Can you work these out from the model? Positions are in its coordinate system, mm. Face numbers are marked on the shaded views. A direction names the side the tool comes from. Round coordinates to 2 decimals unless told otherwise and drop trailing zeros. Loops run counter-clockwise (first coordinate to the right, second up) from the corner with the lowest first, then second, coordinate; pieces in that order, holes last.
(1) I want a section at D-D on y = 15. Write out the boundary of the cut face in (x, z), plus the area to 3 significant figures.
(2) Which directions (+Z, -Z, +X, -X, +Y, -Y) give clear straight access to the entire face, cutting with the end or side of a thin tool? Please do the marked faces 4, 5 and 6.
(3) If I drill on line 1 along Z through (x, y) = (14.5, 14.8); line 2 along Z through (x, y) = (9, 11.5); line 3 along X through (y, z) = (15.35, 0), over which ranges is the centre line in solid material (lowest first)?
(4) I want a section at C-C on y = 10.25. Write out the boundary of the cut face in (x, z), plus the area to 3 significant figures.
(5) I want a section at A-A on x = 33.5. Write out the boundary of the cut face in (y, z).
(6) Thinking about a two-plate mould opening in Y: for the marked faces 1, 2 and 3, which applies, released by +Y, released by -Y, zero draft, split by the parting line, or undercut?
(7) Will these pins go through, and if not, where does the flat tip stop? pin 1 Ø1.5 at (y, z) = (20.5, 12.5) entering from -X; pin 2 Ø10 at (y, z) = (7, -0.5) entering from -X; pin 3 Ø3.5 at (y, z) = (16, 0) entering from +X; pin 4 Ø0.6 at (x, z) = (49, -0.5) entering from +Y.
(8) I want a section at B-B on z = -8. Write out the boundary of the cut face in (x, y), plus the area to 3 significant figures.
Autodesk Inventor part; units mm, degrees
ref_plane "YZ Plane" through (0, 0, 0) normal (1, 0, 0) x (0, 1, 0)
ref_plane "XZ Plane" through (0, 0, 0) normal (0, 1, 0) x (-1, 0, 0)
ref_plane "XY Plane" through (0, 0, 0) normal (0, 0, 1) x (1, 0, 0)
sketch "Sketch1" plane through (0, 0, 0) normal (0, 0, 1) x (1, 0, 0)
  line L0 (0, 0) -> (50, 0)
  line L1 (50, 0) -> (50, 8.5)
  arc A0 (50, 8.5) -> (43.9926, 24) centre (27, 8.5) ccw
  line L2 (43.9926, 24) -> (0, 24)
  line L3 (0, 24) -> (0, 0)
  dimension "d3" = 50
  dimension "d4" = 24
  dimension "d5" = 23
  dimension "d6" = 8.5
extrude "Extrusion1" add sketch "Sketch1" along normal mid plane 39
sketch "Sketch2" plane through (0, 0, 0) normal (0, 0, 1) x (1, 0, 0)
  line L0 (0, 0) -> (0, 24)
  line L1 (0, 13.7) -> (38, 13.7)
  arc A0 (38, 5.7) -> (38, 13.7) centre (38, 9.7) ccw
  line L2 (38, 5.7) -> (24, 5.7)
  line L3 (24, 5.7) -> (24, 0)
  line L4 (50, 0) -> (0, 0)
  line L5 (24, 0) -> (0, 0)
  line L6 (0, 0) -> (0, 13.7)
  dimension "d9" = 5.7
  dimension "d10" = 26
  dimension "d11" = 4
  dimension "d12" = 38
extrude "Extrusion2" cut sketch "Sketch2" along normal mid plane 31
sketch "Sketch3" plane through (0, 0, 0) normal (0, 0, 1) x (1, 0, 0)
  line L0 (0, 24) -> (43.9926, 24)
  line L1 (8, 24) -> (8, 18.2)
  line L2 (8, 18.2) -> (22, 18.2)
  line L3 (22, 18.2) -> (22, 0)
  line L4 (50, 0) -> (0, 0)
  line L5 (45, 0) -> (48, 8.5)
  line L6 (48, 8.5) -> (50, 8.5)
  line L7 (50, 8.5) -> (50, 0)
  line L8 (50, 24) -> (50, 8.5)
  line L9 (8, 24) -> (50, 24)
  line L10 (0, 13.7) -> (38, 13.7)
  dimension "d15" = 4.5
  dimension "d16" = 5
  dimension "d17" = 2
  dimension "d19" = 8.5
  dimension "d20" = 42
  dimension "d31" = 28
extrude "Extrusion3" cut sketch "Sketch3" along normal mid plane 13 contours L0 L9 L8 L6 L5 L4 L3 L2 L1
fillet "Fillet1" radius 6.5 2 edges at (8, 21.1, 6.5) (8, 21.1, -6.5)
sketch "Sketch4" plane through (22, 18.2, 6.5) normal (0, 1, 0) x (1, 0, 0)
  arc A0 (-7.5, 13) -> (-7.5, 0) centre (-7.5, 6.5) ccw
  point P0 (-22, 6.5)
hole "Hole1" at (14.5, 18.2, 0) direction (0, -1, 0) diameter 5.2 end through all countersink diameter 9.5 countersink angle 90
chamfer "Chamfer1" distance 4 angle 45 3 edges at (0, 24, 0) (21.9963, 24, -19.5) (21.9963, 24, 19.5)
properties material "Steel, Carbon"
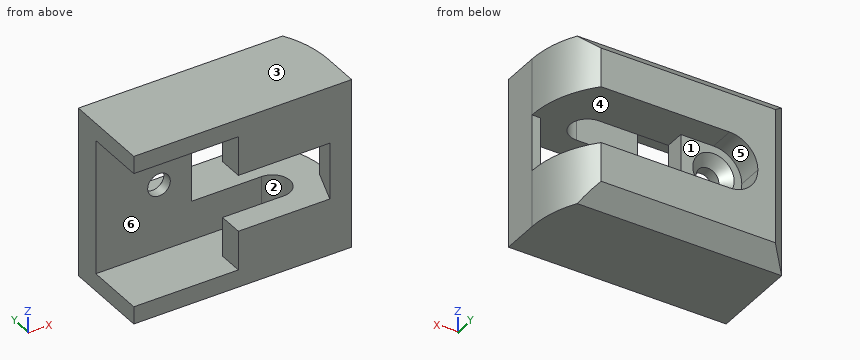
Filled sheet:
1. outline: (0, -19.5) - (49.06, -19.5) - (49.06, -6.5) - (22, -6.5) - (22, 6.5) - (49.06, 6.5) - (49.06, 19.5) - (0, 19.5) - close; hole circle Ø5.2 at (14.5, 0)
1. area: 1,540 mm2
2. face 4: +Y
2. face 5: +X, +Y
2. face 6: -X
3. line 1: z = -19.5 to -2.6, 2.6 to 19.5
3. line 2: z = -19.5 to -15.5, 15.5 to 19.5
3. line 3: x = 0 to 11.9, 17.1 to 22
4. outline: (0, -19.5) - (49.93, -19.5) - (49.93, -6.5) - (41.96, -6.5) - (41.96, -15.5) - (0, -15.5) - close; (0, 15.5) - (41.96, 15.5) - (41.96, 6.5) - (49.93, 6.5) - (49.93, 19.5) - (0, 19.5) - close
4. area: 543 mm2
5. outline: (0, -19.5) - (20, -19.5) - (24, -15.5) - (24, -6.5) - (13.7, -6.5) - (13.7, -15.5) - (5.7, -15.5) - (5.7, -6.5) - (0, -6.5) - close; (0, 6.5) - (5.7, 6.5) - (5.7, 15.5) - (13.7, 15.5) - (13.7, 6.5) - (24, 6.5) - (24, 15.5) - (20, 19.5) - (0, 19.5) - close
6. face 1: released by +Y
6. face 2: undercut
6. face 3: zero draft
7. pin 1: stops at x = 0
7. pin 2: stops at x = 45.71
7. pin 3: stops at x = 22
7. pin 4: stops at y = 8.5
8. outline: (0, 13.7) - (38, 13.7) arc R4 cw to (38, 5.7) - (24, 5.7) - (24, 0) - (50, 0) - (50, 8.5) arc R23 ccw to (43.99, 24) - (4, 24) - (0, 20) - close
8. area: 697 mm2
